Build history of the part. All positions in model axes, mm. A direction names the side the tool comes from. Give positions to 0.01 mm unless a question says otherwise; leave off trailing zeros. Order: outer loops, then holes, each group sorted by start corner. A loop starts at its lowest first (then second) coordinate and runs counter-clockwise, first axis right, second up. Notation, with made-up numbers: (-25, -28) - (4, -28) arc R5 cw to (4, -20) - close; hole circle Ø1 at (5.5, 88.25). An arc over 180 degrees is marked (long way). Answer in a Markdown table with one row per item.
```python
from build123d import *

# Parameters (mm, degrees)
SKETCH2_R          = 9.1
SKETCH2_R_2        = 7.9
CUT_EXTRUDE1_DEPTH = 0.1
CHAMFER1_SIZE      = 1


with BuildPart() as part:
    # Sketch1 → Revolve1 (revolve)
    with BuildSketch(Plane(origin=(0, 0, 0), x_dir=(0, 0, -1), z_dir=(1, 0, 0))):
        Polygon((0, 20.05), (11, 20.05), (11, 14.25), (9.5, 14.25), (9.5, 3.2), (8.75, 3.2), (8.75, 0), (0, 0), align=None)
    revolve(axis=Axis((0, 0, 0), (0, 1, 0)))

    # Sketch2 → Cut-Extrude1 (cut)
    with BuildSketch(Plane(origin=(0, 20.05, 0), x_dir=(1, 0, 0), z_dir=(0, 1, 0))):
        with Locations(Location((0, 0, 0), (0, 0, 270))):
            Circle(SKETCH2_R)
        with Locations(Location((0, 0, 0), (0, 0, 270))):
            Circle(SKETCH2_R_2, mode=Mode.SUBTRACT)
    extrude(amount=-CUT_EXTRUDE1_DEPTH, mode=Mode.SUBTRACT)

    # Chamfer1
    chamfer1_edges = [part.edges().sort_by_distance(p)[0] for p in [
        (0, 20.05, 11),
    ]]
    chamfer(chamfer1_edges, length=CHAMFER1_SIZE)


solid = part.part
```
1. Probe line 1 (X direction, y = 20, z = 0); line 2 (Y direction, x = -5, z = -6.75); line 3 (Z direction, x = -2.5, y = 1). List the from-to ranges inside material, lowest first.
Check result:
| item | result |
|---|---|
| line 1 | x = -10.05 to -9.1, -7.9 to 7.9, 9.1 to 10.05 |
| line 2 | y = 0 to 19.95 |
| line 3 | z = -8.39 to 8.39 |
2. Which spindle directions (+Z, -Z, +X, -X, +Y, -Y) get a long thin tool onto all of the face, cutting with end or side? Do faces 1 (the face through (0, 0, 0)), 2 (the face through (5.324, 1.578, 6.944)). Say none if no direction does.
Check result:
| item | result |
|---|---|
| face 1 | +Z, -Z, +X, -X, -Y |
| face 2 | -Y |
3. Two-plate mould, pull along X, no slides. Class faces 3 (the face through (10.74, 16.62, 2.38)), 4 (the face through (4, 19.95, -7)), 5 (the face through (8.1, 20.05, -4.5)): +X half, -X half, draft (parallel to the pull), parting line (faces both ways), or undercut.
Check result:
| item | result |
|---|---|
| face 3 | parting line |
| face 4 | undercut |
| face 5 | draft |
4. Drop flat-ended pins along their axis: P1, Ø1.5, axis at x = 3.5, z = -7.5, coming from the -Y side; P2, Ø4, axis at x = -7, y = 6.5, coming from the -Z side; P3, Ø6, axis at y = 8, z = 3, coming from the -X side; P4, Ø4, axis at y = 4, z = -6, coming from the -X side. Give the stop position or say it passes through.
Check result:
| item | result |
|---|---|
| P1 | stops at y = 0 |
| P2 | stops at z = -8.08 |
| P3 | stops at x = -9.5 |
| P4 | stops at x = -8.62 |
5. Cut at C-C on y = 3.5. Write the cut outline in (x, z).
Check result:
| item | result |
|---|---|
| outline | circle Ø19 at (0, 0) |
6. Cut at B-B on z = 0. Write the cut outline in (x, y), and give its area (3 significant figures).
Check result:
| item | result |
|---|---|
| outline | (-11, 14.25) - (-9.5, 14.25) - (-9.5, 3.2) - (-8.75, 3.2) - (-8.75, 0) - (8.75, 0) - (8.75, 3.2) - (9.5, 3.2) - (9.5, 14.25) - (11, 14.25) - (11, 19.05) - (10, 20.05) - (9.1, 20.05) - (9.1, 19.95) - (7.9, 19.95) - (7.9, 20.05) - (-7.9, 20.05) - (-7.9, 19.95) - (-9.1, 19.95) - (-9.1, 20.05) - (-10, 20.05) - (-11, 19.05) - close |
| area | 392 mm² |
7. Cut at A-A on x = 0. Write the cut outline in (y, z), and give its area (3 significant figures).
Check result:
| item | result |
|---|---|
| outline | (0, -8.75) - (3.2, -8.75) - (3.2, -9.5) - (14.25, -9.5) - (14.25, -11) - (19.05, -11) - (20.05, -10) - (20.05, -9.1) - (19.95, -9.1) - (19.95, -7.9) - (20.05, -7.9) - (20.05, 7.9) - (19.95, 7.9) - (19.95, 9.1) - (20.05, 9.1) - (20.05, 10) - (19.05, 11) - (14.25, 11) - (14.25, 9.5) - (3.2, 9.5) - (3.2, 8.75) - (0, 8.75) - close |
| area | 392 mm² |
